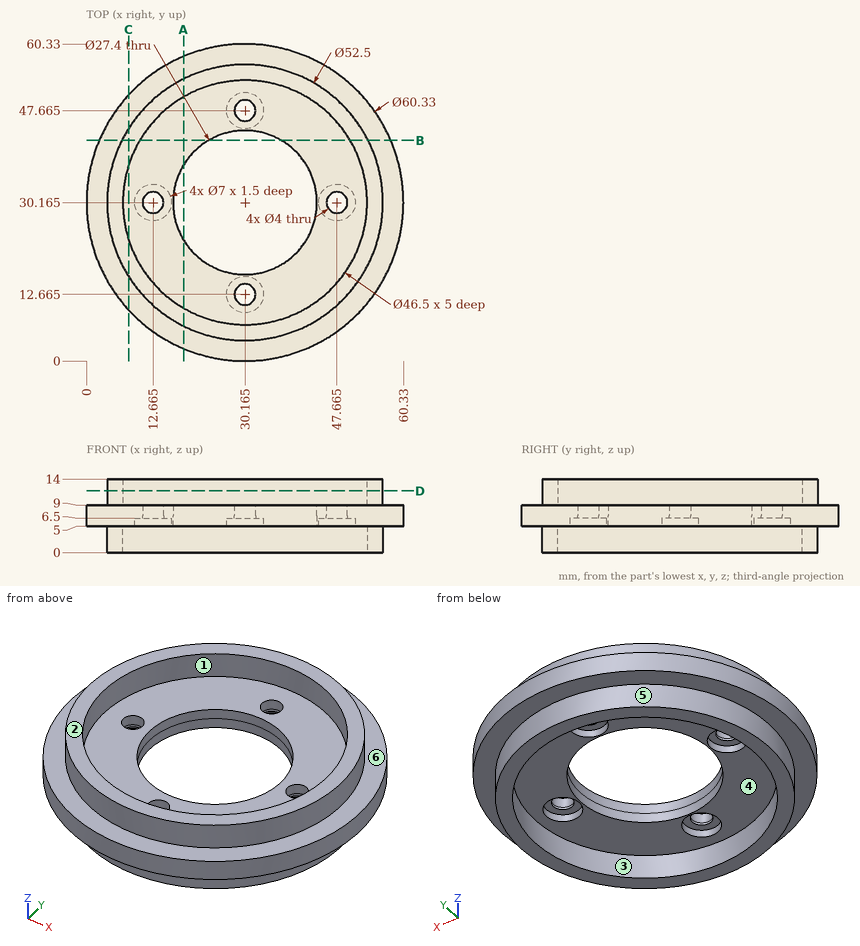
Can you work these out from the drawing? Everything is in mm from the part's minimum corner. A direction names the side the tool comes from. Give positions to 0.01 mm unless a question says otherwise; leave off trailing zeros. Order: outer loops, then holes, each group sorted by start corner. A loop starts at its lowest first (then second) coordinate and runs counter-clockwise, first axis right, second up. Notation, with made-up numbers: (59.5, -3.75) -> (67.5, -3.75) arc R14 ccw to (67.5, 18.25) -> close; hole circle Ø9 at (51.25, 67.5). An arc over 180 degrees is marked (long way). Return JSON: item names as keys, results as strings.
1. Imagine slicing it at D-D on z = 11.75. List the corners of the cut face in (x, y) for me (3 decimals).
Answer list:
{"outline": "circle Ø52.5 at (30.165, 30.165); hole circle Ø46.5 at (30.165, 30.165)"}
2. Imagine slicing it at C-C on x = 8. List the corners of the cut face in (y, z) for me.
Answer list:
{"outline": "(9.7, 5) -> (16.1, 5) -> (16.1, 0) -> (23.15, 0) -> (23.15, 5) -> (37.18, 5) -> (37.18, 0) -> (44.23, 0) -> (44.23, 5) -> (50.63, 5) -> (50.63, 9) -> (44.23, 9) -> (44.23, 14) -> (37.18, 14) -> (37.18, 9) -> (23.15, 9) -> (23.15, 14) -> (16.1, 14) -> (16.1, 9) -> (9.7, 9) -> close"}
3. On a 3-axis mill with a long thin cutter (end or side, diameter ignored), from which of +Z, -Z, +X, -X, +Y, -Y can I reach the whole of each face in a straight line? I mean the marked faces 1, 2 and 3. Say none if no direction works.
Answer list:
{"face 1": "+Z", "face 2": "+Z, +X, -X, +Y, -Y", "face 3": "-Z"}
4. For pin 1 Ø6.5 at (x, y) = (12.665, 30.165) entering from -Z; pin 2 Ø2 at (x, y) = (22.5, 51) entering from +Z; pin 3 Ø3 at (y, z) = (23.5, 12) entering from -X; pin 4 Ø3 at (x, y) = (10, 40) entering from +Z, each with a flat end and sliding along its axis, tell me the tip position at first contact or that it passes through.
Answer list:
{"pin 1": "stops at z = 6.5", "pin 2": "stops at z = 9", "pin 3": "stops at x = 4.43", "pin 4": "stops at z = 14"}
5. Imagine slicing it at A-A on x = 18.5. List the corners of the cut face in (y, z) for me, then the cut area to 3 significant figures.
Answer list:
{"outline": "(2.35, 5) -> (6.65, 5) -> (6.65, 0) -> (10.05, 0) -> (10.05, 5) -> (22.98, 5) -> (22.98, 9) -> (10.05, 9) -> (10.05, 14) -> (6.65, 14) -> (6.65, 9) -> (2.35, 9) -> close; (37.35, 5) -> (50.28, 5) -> (50.28, 0) -> (53.68, 0) -> (53.68, 5) -> (57.98, 5) -> (57.98, 9) -> (53.68, 9) -> (53.68, 14) -> (50.28, 14) -> (50.28, 9) -> (37.35, 9) -> close", "area": "233 mm2"}
6. Imagine slicing it at B-B on y = 42. List the corners of the cut face in (x, z) for me.
Answer list:
{"outline": "(2.42, 5) -> (6.73, 5) -> (6.73, 0) -> (10.15, 0) -> (10.15, 5) -> (23.26, 5) -> (23.26, 9) -> (10.15, 9) -> (10.15, 14) -> (6.73, 14) -> (6.73, 9) -> (2.42, 9) -> close; (37.07, 5) -> (50.18, 5) -> (50.18, 0) -> (53.6, 0) -> (53.6, 5) -> (57.91, 5) -> (57.91, 9) -> (53.6, 9) -> (53.6, 14) -> (50.18, 14) -> (50.18, 9) -> (37.07, 9) -> close"}
7. Thinking about a two-plate mould opening in X: for the marked faces 4, 5 and 6, which applies, pulls with the +X half, pulls with the -X half, needs draft (parallel to the pull), parting line crosses it, or undercut?
Answer list:
{"face 4": "undercut", "face 5": "parting line crosses it", "face 6": "needs draft"}
8. I need wall thicknesses on line 1 (X direction, y = 30, z = 1.75); line 2 (Z direction, x = 18.5, y = 22); line 3 (Y direction, x = 27.5, z = 13.25). Which ranges of each line are inside material? Lowest first, please. Write a range as from..to.
Answer list:
{"line 1": "x = 3.92..6.92, 53.41..56.41", "line 2": "z = 5..9", "line 3": "y = 4.05..7.07, 53.26..56.28"}
